```python
from build123d import *

# Parameters (mm, degrees)
SKETCH1_RX         = 60.325
SKETCH1_RY         = 44.45
BASE_EXTRUDE_DEPTH = 3.175


with BuildPart() as part:
    # Sketch1 → Base-Extrude (new body)
    with BuildSketch(Plane.XY):
        with BuildLine():
            Line((-752.475, -104.363036769), (-679.6278, -367.521079599))
            ThreePointArc((-679.6278, -367.521079599), (0, -273.05), (679.6278, -367.521079599))
            Line((679.6278, -367.521079599), (752.475, -104.363036769))
            ThreePointArc((752.475, -104.363036769), (0, 0), (-752.475, -104.363036769))
        make_face()
        with Locations(Location((-59.197924106, -161.431165366), (0, 0, -95.79))):
            Ellipse(SKETCH1_RX, SKETCH1_RY, mode=Mode.SUBTRACT)
        with Locations(Location((59.197924106, -161.431165366), (0, 0, -84.21))):
            Ellipse(SKETCH1_RX, SKETCH1_RY, mode=Mode.SUBTRACT)
    extrude(amount=-BASE_EXTRUDE_DEPTH)


solid = part.part
```
Build history of the part. All positions in model axes, mm. Round coordinates to 2 decimals unless told otherwise and drop trailing zeros. Order: outer loops, then holes, each group sorted by start corner. A loop starts at its lowest first (then second) coordinate and runs counter-clockwise, first axis right, second up. Notation, with made-up numbers: (20, 28) - (70, 28) arc R21 cw to (70, 59) - close; hole circle Ø9 at (49, 15). An arc over 180 degrees is marked (long way). Use a Markdown table: item, result.
1) Saw through at B-B on y = -175. Give the number of separate pieces and of enclosed holes in the cut face, and give its area (3 significant figures).
Recorded:
| item | result |
|---|---|
| separate pieces | 3 |
| enclosed holes | 0 |
| area | 4,100 mm² |
2) Flat gauge pin, fed straight in: pin 1 Ø5 at (x, y) = (-163.5, -241) entering from +Z. Where does the tip first touch, or does it go through?
Recorded:
| item | result |
|---|---|
| pin 1 | stops at z = 0 |
3) Saw through at A-A on y = -311.5. Write the cut outline in (x, z) (3 decimals).
Recorded:
| item | result |
|---|---|
| outline | (-695.136, -3.175) - (-436.058, -3.175) - (-436.058, 0) - (-695.136, 0) - close; (436.058, -3.175) - (695.136, -3.175) - (695.136, 0) - (436.058, 0) - close |
4) Wall check: L1, parallel to X at y = -175.5, z = -0.35; L2, parallel to X at y = -185, z = -1.4; L3, parallel to Y at x = -92.5, z = -0.4. Give the ranges that are in metal, low to high.
Recorded:
| item | result |
|---|---|
| L1 | x = -732.78 to -103.17, -16.53 to 16.53, 103.17 to 732.78 |
| L2 | x = -730.15 to -101.28, -19.29 to 19.29, 101.28 to 730.15 |
| L3 | y = -274.77 to -204.22, -124.22 to -1.55 |
5) Saw through at C-C on x = 134.5. Write the cut outline in (y, z) (1 decimal).
Recorded:
| item | result |
|---|---|
| outline | (-276.7, -3.2) - (-3.3, -3.2) - (-3.3, 0) - (-276.7, 0) - close |
6) Pull direction X, two halves, no side cores. Call faces 1 (the face through (-9.64, -273.07, -1.57)), 2 (the face through (-716.56, -234.1, -1.57)), 3 (the face through (-11, -181, -3.175)), 4 (the face through (715.541, -237.784, -1.565)): pulls with the +X half, pulls with the -X half, needs draft (parallel to the pull), parting line crosses it, or undercut.
Recorded:
| item | result |
|---|---|
| face 1 | undercut |
| face 2 | pulls with the -X half |
| face 3 | needs draft |
| face 4 | pulls with the +X half |
